For this review, take the finished solid that the model builds, in its own axes (mm). Face numbers are marked on the shaded views. A direction names the side the tool comes from. Coordinates: 2 decimals unless noted, no trailing zeros. Order: outer loops, then holes, each group sorted by start corner. A loop starts at its lowest first (then second) coordinate and runs counter-clockwise, first axis right, second up. Notation, with made-up numbers: (85.25, 72.5) -> (89.25, 72.5) arc R18 ccw to (89.25, 82.5) -> close; hole circle Ø10 at (-23.75, 2). An arc over 180 degrees is marked (long way). Return JSON: item names as keys, results as strings. Group by question number.
Item 1: Take a section at D-D (x = -19). Write out the cut boundary in (y, z) (3 decimals).
Item 2: Take a section at A-A (y = 3.75). Write out the cut boundary in (x, z) (1 decimal), then the cut area to 3 significant figures.
Item 3: Take a section at C-C (z = 0.5). Write out the cut boundary in (x, y) (3 decimals).
Item 4: Machinability: for the marked faces 4 and 5, which of the approach directions +Z, -Z, +X, -X, +Y, -Y give a long, thin tool a straight path to every point of the face, cutting with its end or side? Answer none if there is none.
Item 5: For line 1 along X through (y, z) = (2.25, 2.75) (3 decimals); line 2 along X through (y, z) = (1, -0.75) (3 decimals); line 3 along Z through (x, y) = (11.43, 3.9) (1 decimal), list the stretches that pass through material, from the lowest coordinate up.
Item 6: Insertion check: pin 1 (2.5 mm diameter, centred on x = -11.5, z = 1, fed in from -Y) (3 decimals). The pin has a flat end and moves straight along its axis. Give the tip position at first contact, or say it passes through.
Item 7: Draft analysis for pull direction X (two halves, no side actions). For the marked faces 1, 2 and 3, state which applies: +X half, -X half, draft (parallel to the pull), parting line (faces both ways), or undercut.
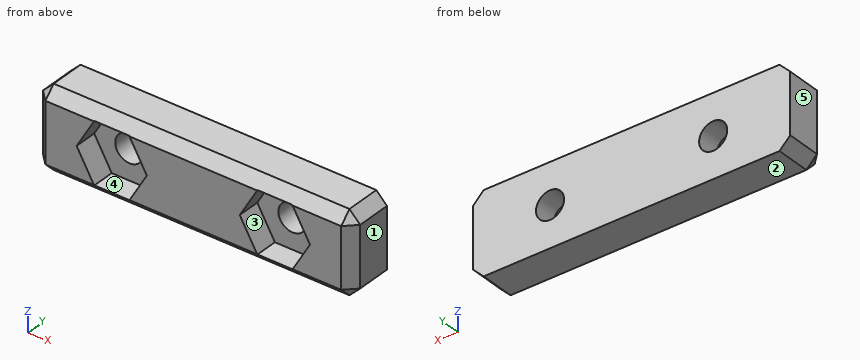
```python
from build123d import *

# Parameters (mm, degrees)
F0_W     = 44.45
F0_H     = 11.43
F1_DEPTH = 6.35
F3_SIZE  = 1.5
F4_DEPTH = 3.175
F5_D     = 3.937
F5_DEPTH = 6.35


with BuildPart() as f1:
    # F0 (on Front) → F1 (new body)
    with BuildSketch(Plane.XZ):
        Rectangle(F0_W, F0_H)
    extrude(amount=-F1_DEPTH)

    # F3
    f3_edges = [f1.edges().sort_by_distance(p)[0] for p in [
        (0, 0, 5.715),
        (0, 0, -5.715),
        (22.225, 0, 0),
        (-22.225, 0, 0),
        (22.225, 3.175, -5.715),
        (22.225, 3.175, 5.715),
        (-22.225, 3.175, 5.715),
        (-22.225, 3.175, -5.715),
    ]]
    chamfer(f3_edges, length=F3_SIZE)

    # F2 (on face) → F4 (cut)
    with BuildSketch(Plane.XZ):
        Polygon((-13.890003, -4.26085), (-8.969997, -4.26085), (-6.509994, 0), (-8.969997, 4.26085), (-13.890003, 4.26085), (-16.350006, 0), align=None)
        Polygon((6.509994, 0), (8.969997, -4.26085), (13.890003, -4.26085), (16.350006, 0), (13.890003, 4.26085), (8.969997, 4.26085), align=None)
    extrude(amount=-F4_DEPTH, mode=Mode.SUBTRACT)

    # F5
    with Locations(Plane.XZ):
        with Locations((-11.43, 0), (11.43, 0)):
            Hole(F5_D / 2, depth=F5_DEPTH)


solid = f1.part
```
Findings below:
{
 "1": {"outline": "(0, -4.215) -> (1.5, -5.715) -> (6.35, -5.715) -> (6.35, 5.715) -> (1.5, 5.715) -> (0, 4.215) -> close"},
 "2": {"outline": "(-22.2, -4.2) -> (-20.7, -5.7) -> (20.7, -5.7) -> (22.2, -4.2) -> (22.2, 4.2) -> (20.7, 5.7) -> (-20.7, 5.7) -> (-22.2, 4.2) -> close; hole circle Ø3.9 at (-11.4, 0); hole circle Ø3.9 at (11.4, 0)", "area": "479 mm2"},
 "3": {"outline": "(-22.225, 1.5) -> (-20.725, 0) -> (-16.061, 0) -> (-16.061, 3.175) -> (-13.334, 3.175) -> (-13.334, 6.35) -> (-22.225, 6.35) -> close; (-9.526, 3.175) -> (-6.799, 3.175) -> (-6.799, 0) -> (6.799, 0) -> (6.799, 3.175) -> (9.526, 3.175) -> (9.526, 6.35) -> (-9.526, 6.35) -> close; (13.334, 3.175) -> (16.061, 3.175) -> (16.061, 0) -> (20.725, 0) -> (22.225, 1.5) -> (22.225, 6.35) -> (13.334, 6.35) -> close"},
 "4": {"face 4": "-Y", "face 5": "+Z, -Z, -X, +Y, -Y"},
 "5": {"line 1": "x = -22.225 to -14.762, -8.098 to 8.098, 14.762 to 22.225", "line 2": "x = -21.725 to -15.917, -6.943 to 6.943, 15.917 to 21.725", "line 3": "z = -5.7 to -2, 2 to 5.7"},
 "6": {"pin 1": "stops at y = 3.175"},
 "7": {"face 1": "+X half", "face 2": "draft", "face 3": "undercut"}
}
